Part model, mm, in its own coordinate system. A direction names the side the tool comes from. Coordinates: 2 decimals unless noted, no trailing zeros. Loops run counter-clockwise (first coordinate to the right, second up) from the corner with the lowest first, then second, coordinate; pieces in that order, holes last. Notation, with made-up numbers: M 33.25,-23 L 53.25,-23 A33 ccw 53.25,16 Z; hole C -39,21 d1. An arc over 180 degrees is marked long. Use a Markdown table: item, result. Add a question column.
1) Wall check: probe 1 along X at (y, z) = (0, 11.25); probe 2 along Y at (x, z) = (13.8, 6); probe 3 along X at (y, z) = (11.5, 8.75). Give the ranges that are in metal, low to high. Write a range as from..to.
2) Band-saw the part on D-D (x = 23.5). List the corners of the cut face in (y, z).
3) Band-saw the part on B-B (z = 16.5). List the corners of the cut face in (x, y), plus the area to 3 significant figures.
4) Pull direction Z, two halves, no side cores. Call faces 6 (the flat face through (-14, 3, 12)), 7 (the cylindrical face through (8.7, -3.2, 4.4)), 8 (the flat face through (-13.2, 1, 6)): released by +Z, released by -Z, zero draft, split by the parting line, or undercut.
5) Band-saw the part on A-A (y = 5.5). List the corners of the cut face in (x, z).
6) Pin check, flat tips, straight feed: pin 1 Ø3 at (x, z) = (0.5, 3.5) entering from +Y; pin 2 Ø6 at (x, y) = (20.5, 4.5) entering from +Z; pin 3 Ø3.5 at (y, z) = (1.5, 5) entering from +X; pin 4 Ø0.9 at (x, z) = (24, 16.5) entering from -Y. Stop position of each tip, or through.
7) Tool access for faces 1 (the flat face through (24, 8.206, 12)), 2 (the flat face through (-5.15, 1, 7)), 3 (the flat face through (13, 9, 6)), 4 (the flat face through (-6.333, 0.304, 4.238)), 5 (the flat face through (-8, 3, 12)): list every direction of +Z, -Z, +X, -X, +Y, -Y with a clear straight run to the whole face (end or side of a thin tool).
from build123d import *

# Parameters (mm, degrees)
SKETCH2_W                 = 5
SKETCH2_H                 = 12
BOSS_EXTRUDE1_DEPTH       = 12
BOSS_EXTRUDE1_2_DEPTH     = 12
BOSS_EXTRUDE3_DEPTH       = 25
SKETCH5_W                 = 3
SKETCH5_H                 = 8.8
BOSS_EXTRUDE4_DEPTH       = 12
SKETCH7_W                 = 2
SKETCH7_H                 = 12
BOSS_EXTRUDE5_DEPTH       = 12
SKETCH15_W                = 0.2
SKETCH15_H                = 12
CUT_EXTRUDE2_DEPTH        = 12
SKETCH16_W                = 0.15
SKETCH16_H                = 12
CUT_EXTRUDE3_DEPTH        = 12
FILLET1_R                 = 6
F_4_0MM_DOWEL_HOLE2_D     = 4
FILLET2_R                 = 6
F_4_0MM_DOWEL_HOLE1_D     = 4
F_4_0MM_DOWEL_HOLE1_DEPTH = 26
F_4_0MM_DOWEL_HOLE1_TIP   = 1.201721238
BOSS_EXTRUDE6_DEPTH       = 1
CUT_EXTRUDE4_DEPTH        = 2.4


with BuildPart() as part:
    # Sketch2 → Boss-Extrude1 (new body)
    with BuildSketch(Plane.XY):
        with Locations((-7.5, 0)):
            Rectangle(SKETCH2_W, SKETCH2_H)
    extrude(amount=BOSS_EXTRUDE1_DEPTH)



with BuildPart() as body_2:
    # Sketch2 → Boss-Extrude1 2 (new body)
    with BuildSketch(Plane.XY):
        with Locations((7.5, 0)):
            Rectangle(SKETCH2_W, SKETCH2_H)
    extrude(amount=BOSS_EXTRUDE1_2_DEPTH)


with BuildPart() as part_1:
    add(part.part)

    add(body_2.part)  # Boss-Extrude3 merges body 2
    # Sketch4 → Boss-Extrude3 (add)
    with BuildSketch(Plane.XY):
        Polygon((-10, 6), (-20, 6), (-22.901603942, 7.206366686), (-26, 7.206366686), (-26, 8.206366686), (-22.7020064, 8.206366686), (-19.800402458, 7), (-10, 7), (10, 7), (19.800402458, 7), (22.7020064, 8.206366686), (26, 8.206366686), (26, 7.206366686), (22.901603942, 7.206366686), (20, 6), (10, 6), align=None)
    extrude(amount=BOSS_EXTRUDE3_DEPTH)

    # Sketch5 → Boss-Extrude4 (add)
    with BuildSketch(Plane.XY):
        with Locations((-11.5, 11.4)):
            Rectangle(SKETCH5_W, SKETCH5_H)
        with Locations((11.5, 11.4)):
            Rectangle(SKETCH5_W, SKETCH5_H)
    extrude(amount=BOSS_EXTRUDE4_DEPTH)

    # Sketch7 → Boss-Extrude5 (add)
    with BuildSketch(Plane.XY):
        with Locations((-14, 0)):
            Rectangle(SKETCH7_W, SKETCH7_H)
        with Locations((14, 0)):
            Rectangle(SKETCH7_W, SKETCH7_H)
    extrude(amount=BOSS_EXTRUDE5_DEPTH)

    # Sketch15 → Cut-Extrude2 (cut)
    with BuildSketch(Plane.XZ.offset(6)):
        with Locations((-9.9, 6)):
            Rectangle(SKETCH15_W, SKETCH15_H)
        with Locations((9.9, 6)):
            Rectangle(SKETCH15_W, SKETCH15_H)
        with Locations((-13.1, 6)):
            Rectangle(SKETCH15_W, SKETCH15_H)
        with Locations((13.1, 6)):
            Rectangle(SKETCH15_W, SKETCH15_H)
    extrude(amount=-CUT_EXTRUDE2_DEPTH, mode=Mode.SUBTRACT)

    # Sketch16 → Cut-Extrude3 (cut)
    with BuildSketch(Plane.XZ.offset(6)):
        with Locations((-5.075, 6)):
            Rectangle(SKETCH16_W, SKETCH16_H)
        with Locations((5.075, 6)):
            Rectangle(SKETCH16_W, SKETCH16_H)
    extrude(amount=-CUT_EXTRUDE3_DEPTH, mode=Mode.SUBTRACT)

    # Fillet1
    fillet1_edges = [part_1.edges().sort_by_distance(p)[0] for p in [
        (7.475, -6, 0),
        (7.475, -6, 12),
        (-7.475, -6, 0),
        (-7.475, -6, 12),
        (-14.1, -6, 0),
        (-14.1, -6, 12),
        (14.1, -6, 12),
        (14.1, -6, 0),
    ]]
    fillet(fillet1_edges, radius=FILLET1_R - 0.0001)  # a hair under: the kernel refuses the full size

    # Ø4.0mm Dowel Hole2 (through all)
    with Locations(Plane(origin=(15, 0, 0), x_dir=(0, 0, -1), z_dir=(1, 0, 0))):
        with Locations((-6, -2)):
            Hole(F_4_0MM_DOWEL_HOLE2_D / 2)

    # Fillet2
    fillet2_edges = [part_1.edges().sort_by_distance(p)[0] for p in [
        (-11.5, 15.8, 0),
        (-11.5, 15.8, 12),
        (11.5, 15.8, 0),
        (11.5, 15.8, 12),
    ]]
    fillet(fillet2_edges, radius=FILLET2_R - 0.0001)  # a hair under: the kernel refuses the full size

    # Ø4.0mm Dowel Hole1
    with Locations(Plane(origin=(13, 0, 0), x_dir=(0, 0, -1), z_dir=(1, 0, 0))):
        with Locations((-6, 11.975)):
            Hole(F_4_0MM_DOWEL_HOLE1_D / 2, depth=F_4_0MM_DOWEL_HOLE1_DEPTH)
            with Locations((0, 0, -(F_4_0MM_DOWEL_HOLE1_DEPTH + F_4_0MM_DOWEL_HOLE1_TIP / 2))):  # 118° drill point
                Cone(0, F_4_0MM_DOWEL_HOLE1_D / 2, F_4_0MM_DOWEL_HOLE1_TIP, mode=Mode.SUBTRACT)

    # Sketch14 → Boss-Extrude6 (add)
    with BuildSketch(Plane.XY):
        Polygon((-22.901603942, 7.206366686), (-26, 7.206366686), (-26, 0), (-15, 0), (-15, 6), (-20, 6), align=None)
        Polygon((20, 6), (15, 6), (15, 0), (26, 0), (26, 7.206366686), (22.901603942, 7.206366686), align=None)
    extrude(amount=BOSS_EXTRUDE6_DEPTH)

    # Sketch18 → Cut-Extrude4 (cut)
    with BuildSketch(Plane(origin=(-5.15, 0, 0), x_dir=(0, 0, -1), z_dir=(1, 0, 0))):
        Polygon((-2.918757855, -0.688786755), (-5.594922908, 1.324040596), (-8.676165053, 0.01282735), (-9.081242145, -3.311213245), (-6.405077092, -5.324040596), (-3.323834947, -4.01282735), align=None)
    cut_extrude4 = extrude(amount=-CUT_EXTRUDE4_DEPTH, mode=Mode.SUBTRACT)

    # Mirror1: Cut-Extrude4 across plane
    add(cut_extrude4.mirror(Plane(origin=(0, 0, 0), x_dir=(0, 0, 1), z_dir=(1, 0, 0))), mode=Mode.SUBTRACT)


solid = part_1.part
Entries:
| question | item | result |
|---|---|---|
| 1 | probe 1 | -15..-13.2, -9.8..-5.15, 5.15..9.8, 13.2..15 |
| 1 | probe 2 | -6..-4, 0..7 |
| 1 | probe 3 | -13..-10, 10..13 |
| 2 | outline | M 0,0 L 8.21,0 L 8.21,25 L 7.21,25 L 7.21,1 L 0,1 Z |
| 3 | outline | M -26,7.21 L -22.9,7.21 L -20,6 L 20,6 L 22.9,7.21 L 26,7.21 L 26,8.21 L 22.7,8.21 L 19.8,7 L -19.8,7 L -22.7,8.21 L -26,8.21 Z |
| 3 | area | 52.5 mm2 |
| 4 | face 6 | released by +Z |
| 4 | face 7 | undercut |
| 4 | face 8 | zero draft |
| 5 | outline | M -26,0 L -13.2,0 L -13.2,12 L -15,12 L -15,1 L -26,1 Z; M -9.8,0 L -5.15,0 L -5.15,12 L -9.8,12 Z; M 5.15,0 L 9.8,0 L 9.8,12 L 5.15,12 Z; M 13.2,0 L 26,0 L 26,1 L 15,1 L 15,12 L 13.2,12 Z |
| 6 | pin 1 | y = 7 |
| 6 | pin 2 | z = 25 |
| 6 | pin 3 | x = 15 |
| 6 | pin 4 | y = 7.21 |
| 7 | face 1 | +Z, -Z, +X, +Y |
| 7 | face 2 | +Z, -Z, -Y |
| 7 | face 3 | +Z, -Z, +Y |
| 7 | face 4 | none |
| 7 | face 5 | +Z, +X, -X, -Y |
